from build123d import *

# Parameters (mm, degrees)
F1_DEPTH = 25
F2_R     = 1.75
F3_DEPTH = 25
F4_R     = 1.461251
F5_DEPTH = 25
F6_SIZE  = 2


with BuildPart() as f1:
    # F0 (on Top) → F1 (new body)
    with BuildSketch(Plane.XY):
        Polygon((0, 15), (0, 0), (15, 0), (15, 5), (5, 5), (5, 15), align=None)
    extrude(amount=F1_DEPTH)

    # F2 (on face) → F3 (cut)
    with BuildSketch(Plane.YZ.offset(5)):
        with Locations((10, 6.5)):
            Circle(F2_R)
        with Locations((10, 18.5)):
            Circle(F2_R)
    extrude(amount=-F3_DEPTH, mode=Mode.SUBTRACT)

    # F4 (on face) → F5 (cut)
    with BuildSketch(Plane(origin=(0, 5, 0), x_dir=(-1, 0, 0), z_dir=(0, 1, 0))):
        with Locations((-10, 2.5)):
            Circle(F4_R)
        with Locations((-10, 22.5)):
            Circle(F4_R)
    extrude(amount=-F5_DEPTH, mode=Mode.SUBTRACT)

    # F6
    f6_edges = [f1.edges().sort_by_distance(p)[0] for p in [
        (5, 5, 12.5),
    ]]
    chamfer(f6_edges, length=F6_SIZE)


solid = f1.part
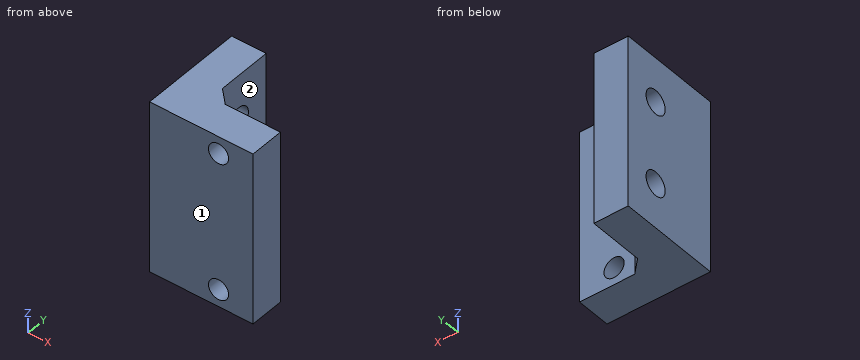
Source: CAD feature listing. Evaluate the final solid. Frame: model axes, mm. Face numbers are marked on the shaded views. A direction names the side the tool comes from. Give positions to 0.01 mm unless a question says otherwise; leave off trailing zeros. Write each loop counter-clockwise with the first axis right and the second up, starting at its lowest first coordinate (ties: lowest second). Pieces come first, ordered by that corner, then holes. Notation, with made-up numbers: M 9.25,74.5 L 60.25,74.5 A21 ccw 60.25,86.5 Z; hole C 4,10 d5. An arc over 180 degrees is marked long. Return JSON: item names as keys, results as strings. Group by question number.
1) Cut plane B-B, the plane z = 18.5. Output: boundary loops of the cut face in (x, y), then the cut area to 4 significant figures.
2) Set-up query: the marked faces 1 and 2. Return all of +Z, -Z, +X, -X, +Y, -Y with unobstructed straight access to the full face (end or side cutting, diameter ignored); none if empty.
3) Cut plane A-A, the plane y = 10. Output: boundary loops of the cut face in (x, z).
4) Cut plane D-D, the plane z = 22.5. Output: boundary loops of the cut face in (x, y), then the cut area to 3 significant figures.
5) Ray query, L1, parallel to Z at x = 10, y = 2.55; L2, parallel to Z at x = 2.8, y = 10; L3, parallel to Y at x = 8.25, z = 14.75. Return the intervals inside material, ascending.
6) First-contact query: pin 1 Ø6 at (y, z) = (5, 6.5) entering from -X; pin 2 Ø6.5 at (x, z) = (9, 17.5) entering from +Y; pin 3 Ø9 at (y, z) = (10, 12) entering from +X; pin 4 Ø3 at (y, z) = (10.5, 7) entering from +X. Flat tips, straight axial feed; report the tip coordinate or a pass-through.
7) Cut plane C-C, the plane x = 10. Output: boundary loops of the cut face in (y, z), then the cut area to 3 significant figures.
Data:
{
 "1": {"outline": "M 0,0 L 15,0 L 15,5 L 7,5 L 5,7 L 5,8.25 L 0,8.25 Z; M 0,11.75 L 5,11.75 L 5,15 L 0,15 Z", "area": "109.5 mm²"},
 "2": {"face 1": "+Z, -Z, +X, -X, -Y", "face 2": "+Z, -Z, +X, +Y"},
 "3": {"outline": "M 0,0 L 5,0 L 5,4.75 L 0,4.75 Z; M 0,8.25 L 5,8.25 L 5,16.75 L 0,16.75 Z; M 0,20.25 L 5,20.25 L 5,25 L 0,25 Z"},
 "4": {"outline": "M 0,0 L 8.54,0 L 8.54,5 L 7,5 L 5,7 L 5,15 L 0,15 Z; M 11.46,0 L 15,0 L 15,5 L 11.46,5 Z", "area": "112 mm²"},
 "5": {"L1": "z = 0 to 1.04, 3.96 to 21.04, 23.96 to 25", "L2": "z = 0 to 4.75, 8.25 to 16.75, 20.25 to 25", "L3": "y = 0 to 5"},
 "6": {"pin 1": "stops at x = 0", "pin 2": "stops at y = 6.25", "pin 3": "stops at x = 6.5", "pin 4": "stops at x = 5"},
 "7": {"outline": "M 0,0 L 5,0 L 5,1.04 L 0,1.04 Z; M 0,3.96 L 5,3.96 L 5,21.04 L 0,21.04 Z; M 0,23.96 L 5,23.96 L 5,25 L 0,25 Z", "area": "95.8 mm²"}
}
